Autodesk Inventor part; units mm, degrees
ref_plane "YZ Plane" through (0, 0, 0) normal (1, 0, 0) x (0, 1, 0)
ref_plane "XZ Plane" through (0, 0, 0) normal (0, 1, 0) x (-1, 0, 0)
ref_plane "XY Plane" through (0, 0, 0) normal (0, 0, 1) x (1, 0, 0)
sketch "Sketch1" plane through (0, 0, 0) normal (0, 0, 1) x (1, 0, 0)
  line L0 (-21.2887, 16.8434) -> (23.7113, 16.8434)
  line L1 (23.7113, 16.8434) -> (23.7113, -34.1566)
  line L2 (23.7113, -34.1566) -> (-21.2887, -34.1566)
  line L3 (-21.2887, -34.1566) -> (-21.2887, 16.8434)
  point P0 (0, 0)
  dimension "d0" = 45
  dimension "d1" = 51
extrude "Extrusion1" add sketch "Sketch1" along normal blind 3.175
sketch "Sketch2" plane through (0, 0, 3.175) normal (0, 0, 1) x (1, 0, 0)
  line L0 (-21.2887, -34.1566) -> (-21.2887, 16.8434)
  line L1 (-21.2887, -34.1566) -> (-21.2887, -9.1566)
  circle A0 centre (-5.2887, -9.1566) radius 8
  circle A1 centre (-13.2887, -9.1566) radius 1
  circle A2 centre (-5.2887, -1.1566) radius 1
  circle A3 centre (2.7113, -9.1566) radius 1
  circle A4 centre (-5.2887, -17.1566) radius 1
  point P0 (0, 0)
  dimension "d4" = 25
  dimension "d6" = 16
  dimension "d7" = 2
  dimension "d8" = 2
  dimension "d9" = 2
  dimension "d10" = 2
  dimension "d11" = 16
extrude "Extrusion2" cut sketch "Sketch2" against normal blind 25.4 contours A0 A3 | A0 A3 | A2 A0 | A0 A2 | A4 A0 | A0 A4 | A1 A0 | A0 A1
sketch "Sketch3" plane through (0, 0, 3.175) normal (0, 0, 1) x (1, 0, 0)
  circle A0 centre (-5.2887, -9.1566) radius 1.9812
  point P0 (0, 0)
  dimension "d14" = 3.9624
extrude "Extrusion3" cut sketch "Sketch3" against normal blind 25.4
sketch "Sketch4" plane through (0, 0, 0) normal (0, 0, -1) x (-1, 0, 0)
  circle A0 centre (5.2887, -9.1566) radius 1.9812
  circle A1 centre (5.2887, -17.1566) radius 1
  circle A2 centre (13.2887, -9.1566) radius 1
  circle A3 centre (5.2887, -1.1566) radius 1
  circle A4 centre (-2.7113, -9.1566) radius 1
  line L0 (21.2887, 16.8434) -> (-23.7113, 16.8434)
  line L1 (-23.7113, 16.8434) -> (-23.7113, -34.1566)
  line L2 (-23.7113, -34.1566) -> (21.2887, -34.1566)
  line L3 (21.2887, -34.1566) -> (21.2887, 16.8434)
  line L4 (-23.7113, -34.1566) -> (-17.3613, -34.1566)
  point P0 (0, 0)
  dimension "d17" = 6.35
extrude "Extrusion4" add sketch "Sketch4" along normal blind 3.175
sketch "Sketch5" plane through (23.7113, -34.1566, 3.175) normal (1, 0, 0) x (0, 0, -1)
  line L0 (0, 51) -> (0, 0)
  line L1 (0, 0) -> (6.35, 0)
  line L2 (6.35, 0) -> (6.35, 51)
  line L3 (0, 51) -> (6.35, 51)
  point P0 (3.175, 34.1566)
extrude "Extrusion5" add sketch "Sketch5" along normal blind 3.175
sketch "Sketch6" plane through (0, 0, 3.175) normal (0, 0, 1) x (1, 0, 0)
  line L0 (-21.2887, 16.8434) -> (26.8863, 16.8434)
  line L1 (26.8863, 16.8434) -> (20.5363, 16.8434)
  line L2 (20.5363, 16.8434) -> (14.1863, 16.8434)
  line L3 (14.1863, 16.8434) -> (14.1863, 4.1434)
  line L4 (14.1863, 4.1434) -> (20.5363, 4.1434)
  line L5 (20.5363, 4.1434) -> (20.5363, 16.8434)
  line L6 (14.1863, 4.1434) -> (20.5363, 4.1434)
  line L7 (20.5363, 4.1434) -> (20.5363, -2.2066)
  line L8 (20.5363, -2.2066) -> (14.1863, -2.2066)
  line L9 (14.1863, -2.2066) -> (14.1863, 4.1434)
  point P0 (0, 0)
  dimension "d22" = 6.35
  dimension "d23" = 6.35
  dimension "d24" = 12.7
  dimension "d25" = 6.35
extrude "Extrusion6" cut sketch "Sketch6" against normal blind 25.4
properties part number "sidebasehole"
The listing builds one solid part. Answer for the finished solid, in the listing's coordinates (mm). A direction names the side the tool comes from. Give positions to 0.01 mm unless a question says otherwise; leave off trailing zeros. Write each loop counter-clockwise with the first axis right and the second up, starting at its lowest first coordinate (ties: lowest second). Pieces come first, ordered by that corner, then holes.
1) Given P1, Ø3, axis at x = -5.29, y = -9.16, coming from the +Z side; P2, Ø6.5, axis at x = -5.29, y = -9.16, coming from the -Z side (3 decimals); P3, Ø1.9, axis at x = 18.5, z = -0.5, coming from the +Y side, each flat-ended and moving along its own axis, determine where each tip first touches the part or whether it passes through.
2) For a pull along X with two mould halves and no side action, classify faces 1 (the face through (20.536, 7, 0)), 2 (the face through (17, -2.207, 0)), 3 (the face through (-3, -8, 3.175)), 4 (the face through (26.886, -8, 0)) as pulls with the +X half, pulls with the -X half, needs draft (parallel to the pull), parting line crosses it, or undercut.
3) Section A-A (z = 2) is taken. Write down the section's boundary in (x, y), and give its area (3 significant figures).
4) Section B-B (x = 19.5) is taken. Write down the section's boundary in (y, z) (3 decimals), and give its area (3 significant figures).
5) Find the intervals of material crossed by L1, parallel to X at y = -1, z = -0.75; L2, parallel to X at y = 7, z = 1.5; L3, parallel to X at y = -1.5, z = 0, in increasing order.
6) A tool of negligible diameter and unlimited length cuts with its end or side. For faces 5 (the face through (-4, 16.843, 0)), 6 (the face through (14.186, 7, 0)), from which of +Z, -Z, +X, -X, +Y, -Y can it reach the whole face along a straight path? Write none if from no direction.
Response:
1. P1: passes through
1. P2: stops at z = -3.175
1. P3: stops at y = -2.21
2. face 1: undercut
2. face 2: undercut
2. face 3: needs draft
2. face 4: pulls with the +X half
3. outline: (-21.29, -34.16) - (26.89, -34.16) - (26.89, 16.84) - (20.54, 16.84) - (20.54, -2.21) - (14.19, -2.21) - (14.19, 16.84) - (-21.29, 16.84) - close; hole circle Ø2 at (-13.29, -9.16); hole circle Ø3.96 at (-5.29, -9.16); hole circle Ø2 at (-5.29, -17.16); hole circle Ø2 at (-5.29, -1.16); hole circle Ø2 at (2.71, -9.16)
3. area: 2,310 mm2
4. outline: (-34.157, -3.175) - (-2.207, -3.175) - (-2.207, 3.175) - (-34.157, 3.175) - close
4. area: 203 mm2
5. L1: x = -21.29 to -6.28, -4.3 to 14.19, 20.54 to 26.89
5. L2: x = -21.29 to 14.19, 20.54 to 26.89
5. L3: x = -21.29 to -6.23, -4.35 to 14.19, 20.54 to 26.89
6. face 5: +Z, -Z, +X, -X, +Y
6. face 6: +Z, -Z, +Y
